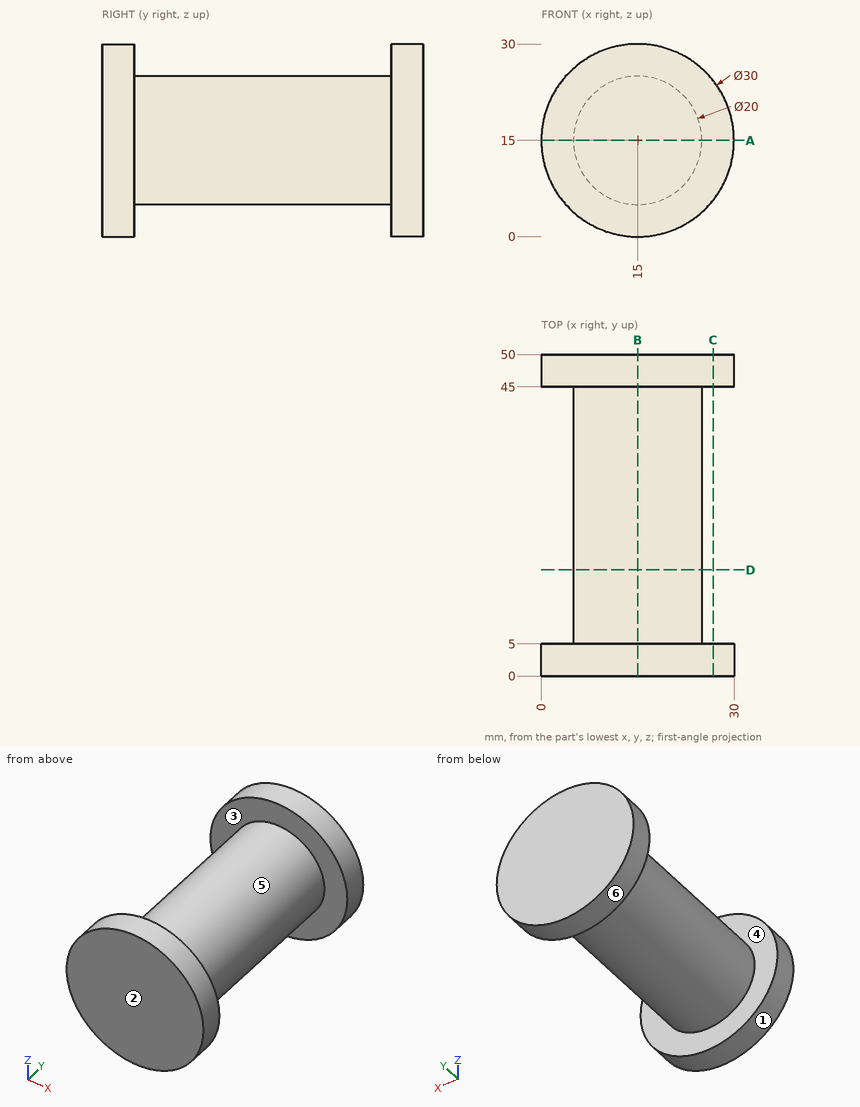
Could you check a few things on this drawing? It's one solid part, dimensions in mm from its lowest x, y, z. A direction names the side the tool comes from. Coordinates: 2 decimals unless noted, no trailing zeros. Order: outer loops, then holes, each group sorted by start corner. A loop starts at its lowest first (then second) coordinate and runs counter-clockwise, first axis right, second up. Notation, with made-up numbers: (43.5, 85.25) -> (64.5, 85.25) arc R27 ccw to (64.5, 103.25) -> close; hole circle Ø3 at (26, -26). An arc over 180 degrees is marked (long way). Answer in a Markdown table with one row per item.
(1) On a 3-axis mill with a long thin cutter (end or side, diameter ignored), from which of +Z, -Z, +X, -X, +Y, -Y can I reach the whole of each face in a straight line? I mean the marked faces 5 and 6. Say none if no direction works.
Answer key:
| item | result |
|---|---|
| face 5 | none |
| face 6 | +Y, -Y |
(2) I want a section at D-D on y = 16.5. List the corners of the cut face in (x, z) for me, then the cut area to 3 significant figures.
Answer key:
| item | result |
|---|---|
| outline | circle Ø20 at (15, 15) |
| area | 314 mm^2 |
(3) Will these pins go through, and if not, where does the flat tip stop? pin 1 Ø1 at (y, z) = (17.5, 18.5) entering from -X; pin 2 Ø8 at (y, z) = (27.5, 18) entering from +X; pin 3 Ø1.5 at (x, y) = (18, 15.5) entering from -Z.
Answer key:
| item | result |
|---|---|
| pin 1 | x = 5.46 |
| pin 2 | x = 25 |
| pin 3 | z = 5.26 |
(4) I want a section at A-A on z = 15. List the corners of the cut face in (x, y) for me.
Answer key:
| item | result |
|---|---|
| outline | (0, 0) -> (30, 0) -> (30, 5) -> (25, 5) -> (25, 45) -> (30, 45) -> (30, 50) -> (0, 50) -> (0, 45) -> (5, 45) -> (5, 5) -> (0, 5) -> close |
(5) Please list where these lines run through material, in increasing order: probe 1 along Y at (x, z) = (8.5, 28.25); probe 2 along Z at (x, y) = (15.5, 27.5); probe 3 along X at (y, z) = (28, 15.25).
Answer key:
| item | result |
|---|---|
| probe 1 | 0 to 5, 45 to 50 |
| probe 2 | 5.01 to 24.99 |
| probe 3 | 5 to 25 |
(6) Thinking about a two-plate mould opening in Y: for the marked faces 1, 2, 3 and 4, which applies, +Y half, -Y half, draft (parallel to the pull), parting line (faces both ways), or undercut?
Answer key:
| item | result |
|---|---|
| face 1 | draft |
| face 2 | -Y half |
| face 3 | undercut |
| face 4 | undercut |
(7) I want a section at C-C on x = 26.75. List the corners of the cut face in (y, z) for me.
Answer key:
| item | result |
|---|---|
| outline | (0, 5.68) -> (5, 5.68) -> (5, 24.32) -> (0, 24.32) -> close; (45, 5.68) -> (50, 5.68) -> (50, 24.32) -> (45, 24.32) -> close |
(8) I want a section at B-B on x = 15. List the corners of the cut face in (y, z) for me.
Answer key:
| item | result |
|---|---|
| outline | (0, 0) -> (5, 0) -> (5, 5) -> (45, 5) -> (45, 0) -> (50, 0) -> (50, 30) -> (45, 30) -> (45, 25) -> (5, 25) -> (5, 30) -> (0, 30) -> close |
